Check sheet for the modelled part. Datum: model origin and axes. Units: mm. A direction names the side the tool comes from. Round coordinates to 2 decimals unless told otherwise and drop trailing zeros. Order: outer loops, then holes, each group sorted by start corner. A loop starts at its lowest first (then second) coordinate and runs counter-clockwise, first axis right, second up.
Q1. Cross-section at D-D on z = 9. Record the cut outline in (x, y).
Q2. Mould release check, pull along X, two halves, no side actions. Record for faces 3 (the flat face through (0, 3.1, 6)), 4 (the flat face through (0, 7, 40)), 5 (the flat face through (5.6, 2, 31)): +X half, -X half, draft (parallel to the pull), parting line (faces both ways), or undercut.
Q3. Depth check by flat-ended pin: P1, Ø1.8, axis at x = 0, y = 7.1, coming from the +Z side; P2, Ø2, axis at x = 0, z = 43, coming from the +Y side; P3, Ø3, axis at x = -2.5, y = 4, coming from the +Z side. Enter the tip coordinate at first touch or a pass-through.
Q4. Scan lines: probe 1 along Y at (x, z) = (4, 18); probe 2 along Z at (x, y) = (1, -9); probe 3 along X at (y, z) = (12, 5). Record each from-to range of solid material in increasing order.
Q5. Cross-section at C-C on y = -8. Record the cut outline in (x, z).
Q6. Set-up check for faces 1 (the cylindrical face through (0.08, -16.51, 47.75)), 2 (the flat face through (-3, 11, 40)): record each of +Z, -Z, +X, -X, +Y, -Y from which the full face is reachable in a straight line by a thin tool's end or side.
Q7. Cross-section at A-A on z = 39. Record the cut outline in (x, y).
Q8. Cross-section at B-B on x = 3. Record the cut outline in (y, z), then the cut area to 3 significant figures.
Autodesk Inventor part; units mm, degrees
ref_plane "YZ Plane" through (0, 0, 0) normal (1, 0, 0) x (0, 1, 0)
ref_plane "XZ Plane" through (0, 0, 0) normal (0, 1, 0) x (-1, 0, 0)
ref_plane "XY Plane" through (0, 0, 0) normal (0, 0, 1) x (1, 0, 0)
ref_plane "Work Plane1" through (0, 0, 0) normal (0, 0, 1) x (1, 0, 0)
sketch "Sketch1" plane through (0, 0, 0) normal (0, 0, 1) x (1, 0, 0)
  circle A0 centre (0, 7.1) radius 1.5
  circle A1 centre (3, 11.1) radius 1.5
  circle A2 centre (-3, 11.1) radius 1.5
  line L0 (-5.8, -25.5252) -> (-5.8, 18.8938)
  line L1 (-5.8, 18.8938) -> (5.8, 18.8938)
  line L2 (5.8, 18.8938) -> (5.8, -25.5252)
  line L3 (-5.6, 3.1) -> (5.6, 3.1)
  line L4 (5.6, 3.1) -> (5.6, 15.1)
  line L5 (5.6, 15.1) -> (-5.6, 15.1)
  line L6 (-5.6, 15.1) -> (-5.6, 3.1)
  line L7 (0, 7.1) -> (0, 6.0369) construction
  point P0 (0, 0)
  dimension "d0" = 0.2
  dimension "d1" = 0.2
  dimension "d3" = 4
  dimension "d4" = 4
  dimension "d10" = 4
  dimension "d11" = 3
  dimension "d12" = 3
extrude "Extrusion1" add sketch "Sketch1" along normal blind 40
sketch "Sketch2" plane through (5.6, 3.1, 0) normal (1, 0, 0) x (0, 0, -1)
  circle A0 centre (-40.6, -11.1) radius 2.05 construction
  line L0 (-40, 0) -> (-40, 12)
  circle A1 centre (-40.6, -11.1) radius 11.1162
  line L1 (-40, 12) -> (-50.2033, -5.5012)
  line L2 (0, 0) -> (-40, 0)
  circle A2 centre (-40.6, -11.1) radius 2.15
  line L3 (-33.0963, -19.3015) -> (-12, 0)
  point P0 (0, -3.1)
  dimension "d7" = 4.3
  dimension "d14" = 12
extrude "Extrusion2" add sketch "Sketch2" against normal up to surface (11.2 mm away)
properties part number "pivot module stalk"
Results found:
1. outline: (-5.6, 3.1) - (5.6, 3.1) - (5.6, 15.1) - (-5.6, 15.1) - close; hole circle Ø3 at (-3, 11.1); hole circle Ø3 at (0, 7.1); hole circle Ø3 at (3, 11.1)
2. face 3: draft
2. face 4: undercut
2. face 5: +X half
3. P1: stops at z = 45.19
3. P2: stops at y = 11.67
3. P3: stops at z = 47.35
4. probe 1: y = -2.39 to 9.98, 12.22 to 15.1
4. probe 2: z = 25.23 to 38.7, 42.5 to 51.67
4. probe 3: x = -5.6 to -4.2, -1.8 to 1.8, 4.2 to 5.6
5. outline: (-5.6, 24.13) - (5.6, 24.13) - (5.6, 38.45) - (-5.6, 38.45) - close; (-5.6, 42.75) - (5.6, 42.75) - (5.6, 51.72) - (-5.6, 51.72) - close
6. face 1: +X, -X
6. face 2: -Z
7. outline: (-5.6, -19) - (5.6, -19) - (5.6, -9.44) - (-5.6, -9.44) - close; (-5.6, -6.56) - (5.6, -6.56) - (5.6, 15.1) - (-5.6, 15.1) - close; hole circle Ø3 at (-3, 11.1); hole circle Ø3 at (0, 7.1); hole circle Ø3 at (3, 11.1)
8. outline: (-16.2, 33.1) - (3.1, 12) - (3.1, 0) - (9.6, 0) - (9.6, 40) - (12.6, 40) - (12.6, 0) - (15.1, 0) - (15.1, 40) - (-2.4, 50.2) arc R11.12 ccw to start; hole circle Ø4.3 at (-8, 40.6)
8. area: 951 mm2
